from build123d import *

# Parameters (mm, degrees)
SKETCH1_R           = 0.5842
SKETCH1_R_2         = 1.8161
SKETCH1_R_3         = 1.6256
SKETCH1_W           = 19.05
SKETCH1_H           = 3.175
BOSS_EXTRUDE2_DEPTH = 3.175


with BuildPart() as part:
    # Sketch1 → Boss-Extrude2 (new body)
    with BuildSketch(Plane(origin=(0, 0, 0), x_dir=(1, 0, 0), z_dir=(0, 1, 0))):
        Polygon((13.611818976, 50.8), (129.54, 50.8), (129.54, 31.75), (126.365, 31.75), (126.365, 27.1526), (124.46, 27.1526), (124.46, 29.36875), (121.681875, 29.36875), (121.681875, 27.1526), (120.015, 27.1526), (120.015, 23.6474), (121.681875, 23.6474), (121.681875, 21.43125), (124.46, 21.43125), (124.46, 23.6474), (126.365, 23.6474), (126.365, 19.05), (129.54, 19.05), (129.54, 0), (0, 0), (-123.973111831, 71.575909488), (-98.573111831, 115.57), align=None)
        with Locations(Location((-8.398663944, 21.566725284, 0), (0, 0, 270))):
            Circle(SKETCH1_R, mode=Mode.SUBTRACT)
        with Locations(Location((-4.549181024, 19.344225284, 0), (0, 0, 270))):
            Circle(SKETCH1_R_2, mode=Mode.SUBTRACT)
        with Locations(Location((-0.699698105, 17.121725284, 0), (0, 0, 270))):
            Circle(SKETCH1_R, mode=Mode.SUBTRACT)
        with Locations(Location((-63.911896428, 46.06498613, 0), (0, 0, 270))):
            Circle(SKETCH1_R_3, mode=Mode.SUBTRACT)
        with Locations(Location((64.77, 7.9375, 0), (0, 0, 270))):
            Circle(SKETCH1_R_3, mode=Mode.SUBTRACT)
        Polygon((-96.113714312, 66.489801459), (-79.61593037, 56.964801459), (-81.20343037, 54.215170802), (-97.701214312, 63.740170802), align=None, mode=Mode.SUBTRACT)
        Polygon((-46.620362486, 37.914801459), (-30.122578543, 28.389801459), (-31.710078543, 25.640170802), (-48.207862486, 35.165170802), align=None, mode=Mode.SUBTRACT)
        with Locations((36.195, 7.9375)):
            Rectangle(SKETCH1_W, SKETCH1_H, mode=Mode.SUBTRACT)
        with Locations((93.345, 7.9375)):
            Rectangle(SKETCH1_W, SKETCH1_H, mode=Mode.SUBTRACT)
    extrude(amount=BOSS_EXTRUDE2_DEPTH)


solid = part.part
Model file for the job. Use its own axes, mm. A direction names the side the tool comes from. Coordinates: 2 decimals unless noted, no trailing zeros. Write each loop counter-clockwise with the first axis right and the second up, starting at its lowest first coordinate (ties: lowest second). Pieces come first, ordered by that corner, then holes. Notation, with made-up numbers: (77.25, 69) - (86.25, 69) arc R5 ccw to (86.25, 76) - close; hole circle Ø10 at (70.5, -20.5). An arc over 180 degrees is marked (long way). Write each question's results on one line, items separated by ' | '. Start each with the question number.
1) 3-axis set-ups, long thin cutter, end or side, ignore diameter. For faces 4 (the face through (-61.119, 1.565, -35.287)), 5 (the face through (-39.843, 1.565, -30.336)): which of +Z, -Z, +X, -X, +Y, -Y reach the whole face in a straight line?
2) Mould opens along X. For faces 1 (the face through (5, 0, -46)), 2 (the face through (-43.27, 1.57, -83.64)), 3 (the face through (-89.337, 1.565, -58.911)) say: pulls with the +X half, pulls with the -X half, needs draft (parallel to the pull), parting line crosses it, or undercut.
3) Cut at C-C (x = -85.5). Write the cut outline in (y, z) (3 decimals), then the cut area to 3 significant figures.
4) Cut at B-B (y = 1.35). Count the separate pieces of the cut face and the enclosed holes in it, then the cut area to 3 significant figures.
5) Cut at D-D (z = -87). Write the cut outline in (x, y) (3 decimals).
6) Flat gauge pins, fed straight in: P1, Ø0.8, axis at x = 123, y = 1.5, coming from the -Z side; P2, Ø1.1, axis at y = 1.5, z = -22, coming from the +X side (3 decimals); P3, Ø1, axis at y = 0.5, z = -68, coming from the +X side. Where does each tip first touch, or does it go through?
7) Cut at A-A (x = 99.5). Write the cut outline in (y, z) (3 decimals), then the cut area to 3 significant figures.
8) Probe line 1 along Z through (x, y) = (33, 2.45) (3 decimals); line 2 along Z through (x, y) = (78, 2.1); line 3 along Z through (x, y) = (-6, 2.65). List the from-to ranges inside material, lowest first. Write a range as from..to.
Returned:
1) face 4: +Z, -X, +Y, -Y | face 5: +Y, -Y
2) face 1: needs draft | face 2: pulls with the +X half | face 3: undercut
3) outline: (0, -108.022) - (3.175, -108.022) - (3.175, -60.362) - (0, -60.362) - close; (0, -56.696) - (3.175, -56.696) - (3.175, -49.363) - (0, -49.363) - close | area: 175 mm^2
4) separate pieces: 1 | enclosed holes: 9 | area: 12,800 mm^2
5) outline: (-115.068, 0) - (-49.088, 0) - (-49.088, 3.175) - (-115.068, 3.175) - close
6) P1: z = -50.8 | P2: x = 126.365 | P3: x = -15.31
7) outline: (0, -50.8) - (3.175, -50.8) - (3.175, -9.525) - (0, -9.525) - close; (0, -6.35) - (3.175, -6.35) - (3.175, 0) - (0, 0) - close | area: 151 mm^2
8) line 1: -50.8..-9.525, -6.35..0 | line 2: -50.8..0 | line 3: -62.12..-20.44, -18.25..-3.46
